Geometry check sheet. Reference: drawing and pictorial views, mm from the part's lowest x, y, z. A direction names the side the tool comes from. Coordinates: 2 decimals unless noted, no trailing zeros. Write each loop counter-clockwise with the first axis right and the second up, starting at its lowest first coordinate (ties: lowest second). Pieces come first, ordered by that corner, then holes.
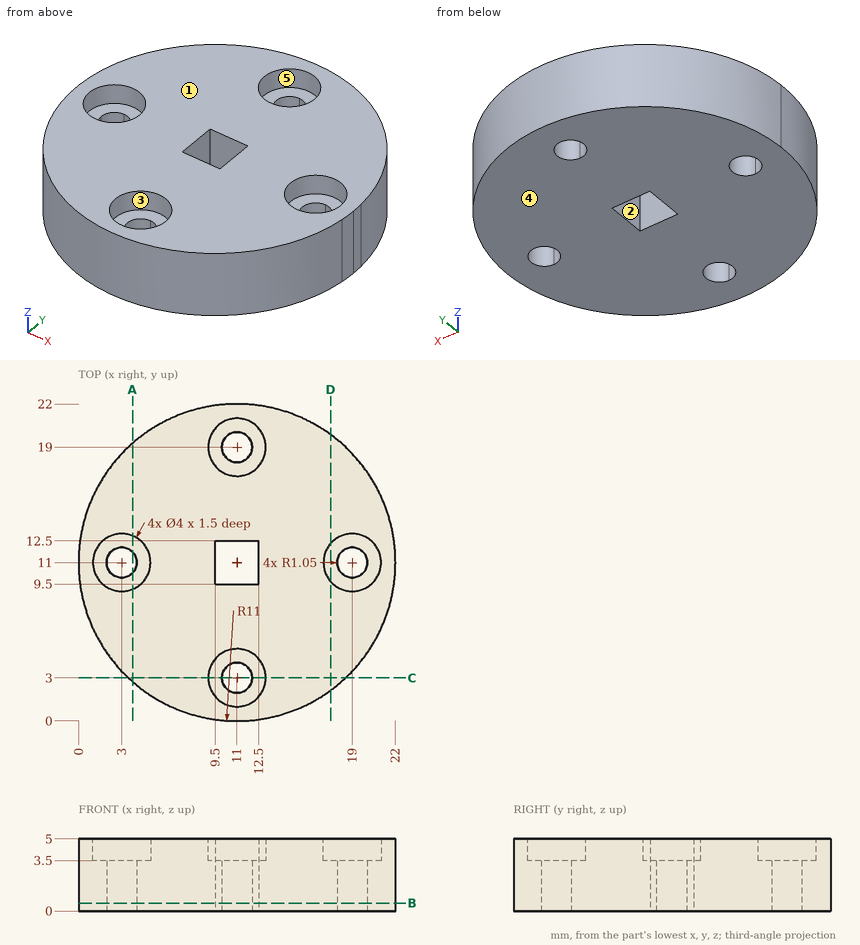
1. Material ranges on L1, parallel to Y at x = 11, z = 3.95; L2, parallel to Y at x = 4.75, z = 0.6; L3, parallel to Y at x = 10.25, z = 3.8, recorded low to high.
2. Tool access check on the marked faces 1, 2 and 3. Record the directions out of +Z, -Z, +X, -X, +Y, -Y that give a thin tool (end or side, any length) a straight path to the whole face; none if there is none.
3. Sectioned sample at A-A, the plane x = 3.75. Record the boundary of the cut face in (y, z), and give its area (3 significant figures).
4. Gauge pin test, flat ends, axial feed: P1, Ø2, axis at x = 9.5, z = 2, coming from the +Y side; P2, Ø1.5, axis at x = 3.5, z = 1, coming from the -Y side; P3, Ø1.5, axis at x = 13, z = 3, coming from the -Y side. Record the tip position at first contact, or that the pin passes through.
5. Draft check along X on the marked faces 4 and 5. Enter one of: pulls with the +X half, pulls with the -X half, needs draft (parallel to the pull), parting line crosses it, or undercut.
6. Sectioned sample at C-C, the plane y = 3. Record the boundary of the cut face in (x, z).
7. Sectioned sample at D-D, the plane x = 17.5. Record the boundary of the cut face in (y, z).
8. Sectioned sample at B-B, the plane z = 0.55. Record the boundary of the cut face in (x, y).
Outcome:
1. L1: y = 0 to 1, 5 to 9.5, 12.5 to 17, 21 to 22
1. L2: y = 1.95 to 20.05
1. L3: y = 0.03 to 1.15, 4.85 to 9.5, 12.5 to 17.15, 20.85 to 21.97
2. face 1: +Z, +X, -X, +Y, -Y
2. face 2: +Z, -Z
2. face 3: +Z
3. outline: (2.73, 0) - (10.27, 0) - (10.27, 3.5) - (9.15, 3.5) - (9.15, 5) - (2.73, 5) - close; (11.73, 0) - (19.27, 0) - (19.27, 5) - (12.85, 5) - (12.85, 3.5) - (11.73, 3.5) - close
3. area: 72.0 mm2
4. P1: stops at y = 21.99
4. P2: stops at y = 2.31
4. P3: stops at y = 0.07
5. face 4: needs draft
5. face 5: undercut
6. outline: (3.45, 0) - (9.95, 0) - (9.95, 3.5) - (9, 3.5) - (9, 5) - (3.45, 5) - close; (12.05, 0) - (18.55, 0) - (18.55, 5) - (13, 5) - (13, 3.5) - (12.05, 3.5) - close
7. outline: (2.13, 0) - (19.87, 0) - (19.87, 5) - (12.32, 5) - (12.32, 3.5) - (9.68, 3.5) - (9.68, 5) - (2.13, 5) - close
8. outline: circle Ø22 at (11, 11); hole circle Ø2.1 at (3, 11); hole (9.5, 9.5) - (12.5, 9.5) - (12.5, 12.5) - (9.5, 12.5) - close; hole circle Ø2.1 at (11, 3); hole circle Ø2.1 at (11, 19); hole circle Ø2.1 at (19, 11)
